Geometry: see drawing. Coordinates: mm, zero at the bounding-box minimum. A direction names the side the tool comes from. Give positions to 0.01 mm unless a question says otherwise; leave off trailing zeros. Write each loop counter-clockwise with the first axis right and the second up, starting at its lowest first coordinate (ties: lowest second). Pieces come first, ordered by that corner, then holes. Notation, with made-up numbers: (48, -17) - (100, -17) arc R6 cw to (100, -12) - close; hole circle Ø5 at (89, -33). An arc over 180 degrees is marked (long way). Use a Markdown table: item, result. Add a question column.
1. Section query C-C, the plane z = 2.35. Return loops of the section in (x, y), plus the area to 3 significant figures.
2. Section query A-A, the plane y = 11. Return loops of the section in (x, z), plus the area to 3 significant figures.
3. Set-up query: the marked faces 1 and 2. Return all of +Z, -Z, +X, -X, +Y, -Y with unobstructed straight access to the full face (end or side cutting, diameter ignored); none if empty.
4. Material intervals for probe 1 along Y at (x, z) = (11, 2.1); probe 2 along Y at (x, z) = (11, 3.9); probe 3 along Z at (x, y) = (16, 3), sorted ascending.
5. Section query D-D, the plane y = 19.75. Return loops of the section in (x, z).
6. Mould query, pull axis Y, two halves, no side actions, for the marked faces 3, 4 and 5. Classes: released by +Y, released by -Y, zero draft, split by the parting line, or undercut.
7. Pin query (flat end, axial travel): pin 1 (1.5 mm diameter, centred on y = 18, z = 1.5, fed in from -X); pin 2 (2 mm diameter, centred on x = 10.5, y = 12, fed in from +Z); pin 3 (1 mm diameter, centred on x = 16, y = 8.5, fed in from -Z); pin 4 (10 mm diameter, centred on x = 7.5, y = 12, fed in from +Z). Return the tip coordinate at first contact, or that it passes through.
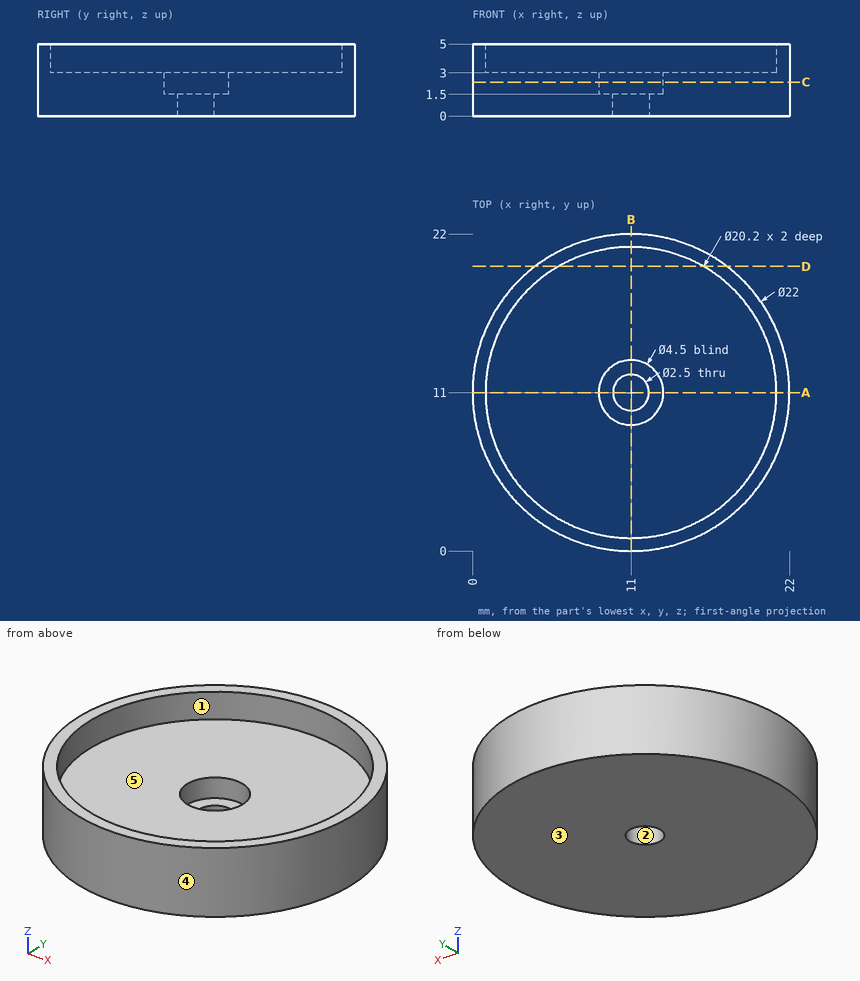
Result sheet:
| question | item | result |
|---|---|---|
| 1 | outline | circle Ø22 at (11, 11); hole circle Ø4.5 at (11, 11) |
| 1 | area | 364 mm² |
| 2 | outline | (0, 0) - (9.75, 0) - (9.75, 1.5) - (8.75, 1.5) - (8.75, 3) - (0.9, 3) - (0.9, 5) - (0, 5) - close; (12.25, 0) - (22, 0) - (22, 5) - (21.1, 5) - (21.1, 3) - (13.25, 3) - (13.25, 1.5) - (12.25, 1.5) - close |
| 2 | area | 59.1 mm² |
| 3 | face 1 | +Z |
| 3 | face 2 | +Z, -Z |
| 4 | probe 1 | y = 0 to 8.75, 13.25 to 22 |
| 4 | probe 2 | y = 0 to 0.9, 21.1 to 22 |
| 4 | probe 3 | z = 0 to 3 |
| 5 | outline | (4.33, 0) - (17.67, 0) - (17.67, 5) - (16.04, 5) - (16.04, 3) - (5.96, 3) - (5.96, 5) - (4.33, 5) - close |
| 6 | face 3 | zero draft |
| 6 | face 4 | split by the parting line |
| 6 | face 5 | undercut |
| 7 | pin 1 | stops at x = 1.95 |
| 7 | pin 2 | stops at z = 1.5 |
| 7 | pin 3 | stops at z = 0 |
| 7 | pin 4 | stops at z = 3 |
